Check sheet for the modelled part. Datum: model origin and axes. Units: mm. Round coordinates to 2 decimals unless told otherwise and drop trailing zeros. Order: outer loops, then holes, each group sorted by start corner. A loop starts at its lowest first (then second) coordinate and runs counter-clockwise, first axis right, second up. Notation, with made-up numbers: M 62.5,11.25 L 74.5,11.25 A13 ccw 74.5,24.25 Z; hole C -5,35.25 d9. An arc over 180 degrees is marked long. One line per item, written item: value. Start each with the question number.
(1) Cross-section at D-D, the plane z = 0.65. Count the separate pieces of the cut face and the enclosed holes in it, and give its area (3 significant figures).
(2) Cross-section at C-C, the plane x = 0. Enter the section's corners in (y, z), and give its area (3 significant figures).
(3) Cross-section at B-B, the plane y = 8.2. Enter the section's corners in (x, z), and give its area (3 significant figures).
(4) Cross-section at A-A, the plane x = 5.66. Enter the section's corners in (y, z), and give its area (3 significant figures).
(5) Thickness scan on L1, parallel to Y at x = 7.66, z = 1.1; L2, parallel to Y at x = 5.66, z = 2.7; L3, parallel to Y at x = 0.5, z = 1.05. Record the ranges inside material, lowest first.
(6) Depth check by flat-ended pin: pin 1 Ø0.8 at (x, y) = (7.66, 8.2) entering from -Z; pin 2 Ø2 at (x, y) = (5.5, 1) entering from -Z. Enter the tip coordinate at first touch or a pass-through.
(7) Release check for a two-part mould opening along Y. For faces 1 (the face through (0, 12.7, 2)), 2 (the face through (10.16, 0, 2)), 3 (the face through (0, -12.7, 2)), 4 (the face through (-0.182, -8.775, 1.878)) record: released by +Y, released by -Y, zero draft, split by the parting line, or undercut.
from build123d import *

# Parameters (mm, degrees)
SKETCH1_W         = 20.32
SKETCH1_H         = 25.4
SKETCH1_R         = 1.397
SKETCH1_R_2       = 0.508
SKETCH1_R_3       = 0.51
BOARD_DEPTH       = 3.81
SKETCH2_W         = 3
SKETCH2_H         = 6
SKETCH2_R         = 0.508
SKETCH2_R_2       = 1.008
SKETCH2_R_3       = 0.81
SKETCH2_R_4       = 0.51
SKETCH2_W_2       = 1.5
SKETCH2_H_2       = 0.4
SKETCH2_W_3       = 0.4
SKETCH2_H_3       = 1.475523652
SOLDER_PADS_DEPTH = 0.1


with BuildPart() as part:
    # Sketch1 → Board (new body)
    with BuildSketch(Plane.XY):
        Rectangle(SKETCH1_W, SKETCH1_H)
        with Locations((0, -10.16)):
            Circle(SKETCH1_R, mode=Mode.SUBTRACT)
        with Locations((0, 1.905)):
            Circle(SKETCH1_R, mode=Mode.SUBTRACT)
        with Locations((-8.66, -3.302)):
            Circle(SKETCH1_R_2, mode=Mode.SUBTRACT)
        with Locations((8.66, -3.302)):
            Circle(SKETCH1_R_2, mode=Mode.SUBTRACT)
        with Locations((-5.66, -3.302)):
            Circle(SKETCH1_R_2, mode=Mode.SUBTRACT)
        with Locations((5.66, -3.302)):
            Circle(SKETCH1_R_2, mode=Mode.SUBTRACT)
        with Locations((7.66, 10.2)):
            Circle(SKETCH1_R_3, mode=Mode.SUBTRACT)
        with Locations((7.66, 8.2)):
            Circle(SKETCH1_R_3, mode=Mode.SUBTRACT)
    extrude(amount=BOARD_DEPTH)

    # Sketch2 → Solder Pads (add)
    with BuildSketch(Plane.XY):
        with Locations((8.66, -3.302)):
            Rectangle(SKETCH2_W, SKETCH2_H)
        with Locations((8.66, -3.302)):
            Circle(SKETCH2_R, mode=Mode.SUBTRACT)
        with Locations((-8.66, -3.302)):
            Rectangle(SKETCH2_W, SKETCH2_H)
        with Locations((-8.66, -3.302)):
            Circle(SKETCH2_R, mode=Mode.SUBTRACT)
        with Locations((5.66, -3.302)):
            Circle(SKETCH2_R_2)
        with Locations((5.66, -3.302)):
            Circle(SKETCH2_R, mode=Mode.SUBTRACT)
        with Locations((-5.66, -3.302)):
            Circle(SKETCH2_R_2)
        with Locations((-5.66, -3.302)):
            Circle(SKETCH2_R, mode=Mode.SUBTRACT)
        with Locations((7.66, 8.2)):
            Circle(SKETCH2_R_3)
        with Locations((7.66, 8.2)):
            Circle(SKETCH2_R_4, mode=Mode.SUBTRACT)
        with Locations((7.66, 10.2)):
            Circle(SKETCH2_R_3)
        with Locations((7.66, 10.2)):
            Circle(SKETCH2_R_4, mode=Mode.SUBTRACT)
        with Locations((7.91, 0.598)):
            Rectangle(SKETCH2_W_2, SKETCH2_H_2)
        with Locations((7.91, 0.575572986)):
            Rectangle(SKETCH2_W_3, SKETCH2_H_3)
        with Locations((-7.91, 0.598)):
            Rectangle(SKETCH2_W_2, SKETCH2_H_2)
    extrude(amount=-SOLDER_PADS_DEPTH)


solid = part.part
Values found:
1. separate pieces: 1
1. enclosed holes: 8
1. area: 499 mm^2
2. outline: M -12.7,0 L -11.56,0 L -11.56,3.81 L -12.7,3.81 Z; M -8.76,0 L 0.51,0 L 0.51,3.81 L -8.76,3.81 Z; M 3.3,0 L 12.7,0 L 12.7,3.81 L 3.3,3.81 Z
2. area: 75.5 mm^2
3. outline: M -10.16,0 L 6.85,0 L 6.85,-0.1 L 7.15,-0.1 L 7.15,3.81 L -10.16,3.81 Z; M 8.17,-0.1 L 8.47,-0.1 L 8.47,0 L 10.16,0 L 10.16,3.81 L 8.17,3.81 Z
3. area: 73.6 mm^2
4. outline: M -12.7,0 L -4.31,0 L -4.31,-0.1 L -3.81,-0.1 L -3.81,3.81 L -12.7,3.81 Z; M -2.79,-0.1 L -2.29,-0.1 L -2.29,0 L 12.7,0 L 12.7,3.81 L -2.79,3.81 Z
4. area: 93.0 mm^2
5. L1: -12.7 to 7.69, 8.71 to 9.69, 10.71 to 12.7
5. L2: -12.7 to -3.81, -2.79 to 12.7
5. L3: -12.7 to -11.46, -8.86 to 0.6, 3.21 to 12.7
6. pin 1: through
6. pin 2: z = 0
7. face 1: released by +Y
7. face 2: zero draft
7. face 3: released by -Y
7. face 4: undercut
